Geometry: final body of the model. Coordinates: model frame, mm. Give positions to 0.01 mm unless a question says otherwise; leave off trailing zeros. Write each loop counter-clockwise with the first axis right and the second up, starting at its lowest first coordinate (ties: lowest second). Pieces come first, ordered by that corner, then holes. Notation, with made-up numbers: (49.25, 78.5) -> (53.25, 78.5) arc R12 cw to (53.25, 88.5) -> close; hole circle Ø10 at (-10.75, 20). An arc over 180 degrees is marked (long way). Answer as a JSON object with one key per item and string values. Group by question number.
(1) Material intervals for probe 1 along Z at (x, y) = (-38, 3); probe 2 along X at (y, z) = (3.25, 39); probe 3 along Z at (x, y) = (-45, 28.5), sorted ascending.
(2) Section query A-A on z = 87. Output: boundary loops of the cut face in (x, y).
(3) Contact query for flat-ended pins moving along their axis: pin 1 Ø6 at (x, y) = (-16.5, 30.5) entering from +Z; pin 2 Ø1.5 at (x, z) = (-38, -81) entering from -Y; pin 3 Ø9.5 at (y, z) = (31.5, 94) entering from -X. Output: stop coordinate, or through.
(4) Section query B-B on x = -10. Output: boundary loops of the cut face in (y, z).
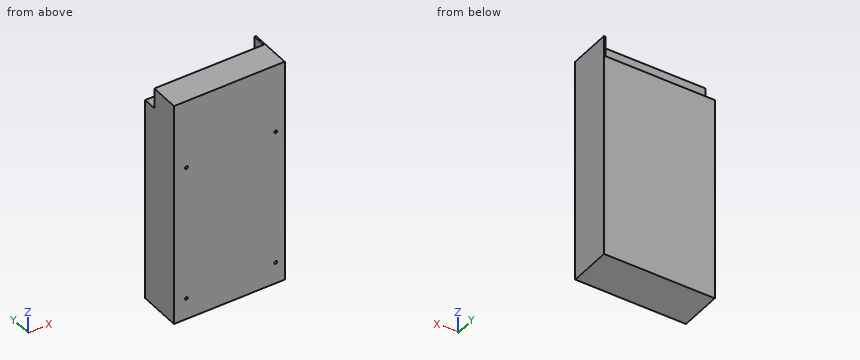
from build123d import *

# Parameters (mm, degrees)
SKETCH_1_W             = 98
SKETCH_1_H             = 200
EXTRUDE_275_DEPTH      = 38
SKETCH_2_W             = 96.5
SKETCH_2_H             = 18
CUT_EXTRUDE_1_DEPTH    = 12
HOLE_WIZARD_M3_1_D     = 2.5
HOLE_WIZARD_M3_1_DEPTH = 5
HOLE_WIZARD_M3_1_TIP   = 0.751075774


with BuildPart() as part:
    # 草图1 → Extrude 275 (new body)
    with BuildSketch(Plane(origin=(0, 0, 0), x_dir=(1, 0, 0), z_dir=(0, 1, 0))):
        Rectangle(SKETCH_1_W, SKETCH_1_H)
    extrude(amount=EXTRUDE_275_DEPTH)

    # 草图2 → 切除-拉伸1 (cut)
    with BuildSketch(Plane(origin=(0, 38, 0), x_dir=(1, 0, 0), z_dir=(0, 1, 0))):
        with Locations((-0.75, -91)):
            Rectangle(SKETCH_2_W, SKETCH_2_H)
    extrude(amount=-CUT_EXTRUDE_1_DEPTH, mode=Mode.SUBTRACT)

    # M3 螺纹孔的螺纹孔钻头1
    with Locations(Plane(origin=(0, 0, 0), x_dir=(-1, 0, 0), z_dir=(0, -1, 0))):
        with Locations((38, -39), (-41, -39), (38, 81), (-41, 81)):
            Hole(HOLE_WIZARD_M3_1_D / 2, depth=HOLE_WIZARD_M3_1_DEPTH)
            with Locations((0, 0, -(HOLE_WIZARD_M3_1_DEPTH + HOLE_WIZARD_M3_1_TIP / 2))):  # 118° drill point
                Cone(0, HOLE_WIZARD_M3_1_D / 2, HOLE_WIZARD_M3_1_TIP, mode=Mode.SUBTRACT)


solid = part.part
Answer list:
{
 "1": {"probe 1": "-100 to -82.25, -79.75 to 37.75, 40.25 to 100", "probe 2": "-49 to -39.25, -36.75 to 39.75, 42.25 to 49", "probe 3": "-100 to 82"},
 "2": {"outline": "(-49, 0) -> (49, 0) -> (49, 38) -> (47.5, 38) -> (47.5, 26) -> (-49, 26) -> close"},
 "3": {"pin 1": "z = 82", "pin 2": "y = 5.3", "pin 3": "x = 47.5"},
 "4": {"outline": "(0, -100) -> (38, -100) -> (38, 82) -> (26, 82) -> (26, 100) -> (0, 100) -> close"}
}
